from build123d import *

# Parameters (mm, degrees)
F1_DEPTH = 70
F2_R     = 5
F4_D     = 4
F4_DEPTH = 10
F4_TIP   = 1.2017212381


with BuildPart() as f1:
    # F0 (on Front) → F1 (new body)
    with BuildSketch(Plane.XZ):
        Polygon((3, 70), (0, 0), (18.5, 0), (18.5, 70), align=None)
    extrude(amount=F1_DEPTH)

    # F2
    f2_edges = [f1.edges().sort_by_distance(p)[0] for p in [
        (18.5, -35, 70),
        (3, -35, 70),
    ]]
    fillet(f2_edges, radius=F2_R)

    # F4
    with Locations(Plane(origin=(0, 0, 0), x_dir=(1, 0, 0), z_dir=(0, 0, -1))):
        with Locations((9.25, 55), (9.25, 15)):
            Hole(F4_D / 2, depth=F4_DEPTH)
            with Locations((0, 0, -(F4_DEPTH + F4_TIP / 2))):  # 118° drill point
                Cone(0, F4_D / 2, F4_TIP, mode=Mode.SUBTRACT)


solid = f1.part
Could you check a few things on this model? Use its own coordinates, in mm. A direction names the side the tool comes from. Give positions to 0.01 mm unless a question says otherwise; leave off trailing zeros. Order: outer loops, then holes, each group sorted by start corner. A loop starts at its lowest first (then second) coordinate and runs counter-clockwise, first axis right, second up.
1. Suppose I cut it at A-A (y = -29). Write out the boundary of the cut face in (x, z).
Answers below:
outline: (0, 0) - (18.5, 0) - (18.5, 65) arc R5 ccw to (13.5, 70) - (7.79, 70) arc R5 ccw to (2.79, 65.21) - close
2. Suppose I cut it at C-C (z = 17.5). Write out the boundary of the cut face in (x, y).
Answers below:
outline: (0.75, -70) - (18.5, -70) - (18.5, 0) - (0.75, 0) - close
3. Suppose I cut it at D-D (z = 53). Write out the boundary of the cut face in (x, y).
Answers below:
outline: (2.27, -70) - (18.5, -70) - (18.5, 0) - (2.27, 0) - close
4. Thinking about a two-plate mould opening in Y: for faces 1 (the flat face through (9, -70, 35)), 2 (the conical face through (9.4, -55.3, 11)), 3 (the cylindrical face through (4.29, -35.49, 68.57)), which applies, +Y half, -Y half, draft (parallel to the pull), parting line (faces both ways), or undercut?
Answers below:
face 1: -Y half
face 2: undercut
face 3: draft
5. For pin 1 (10 mm diameter, centred on y = -59.5, z = 33, fed in from -X); pin 2 (10 mm diameter, centred on x = 7.5, z = 18, fed in from +Y), each with a flat end and sliding along its axis, tell me the tip position at first contact or that it passes through.
Answers below:
pin 1: stops at x = 1.2
pin 2: stops at y = 0
6. Suppose I cut it at B-B (z = 6). Write out the boundary of the cut face in (x, y), plus the area to 3 significant figures.
Answers below:
outline: (0.26, -70) - (18.5, -70) - (18.5, 0) - (0.26, 0) - close; hole circle Ø4 at (9.25, -55); hole circle Ø4 at (9.25, -15)
area: 1,250 mm2
7. I need wall thicknesses on L1, parallel to Y at x = 9.25, z = 3.75; L2, parallel to X at y = -15, z = 6.75; L3, parallel to X at y = -15, z = 3. Which ranges of each line are inside material? Lowest first, please.
Answers below:
L1: y = -70 to -57, -53 to -17, -13 to 0
L2: x = 0.29 to 7.25, 11.25 to 18.5
L3: x = 0.13 to 7.25, 11.25 to 18.5
8. Which directions (+Z, -Z, +X, -X, +Y, -Y) give clear straight access to the entire face, cutting with the end or side of a thin tool? Please do faces 4 (the flat face through (18.5, -35, 32)), 5 (the cylindrical face through (9.51, -56.983, 5.07)).
Answers below:
face 4: +Z, -Z, +X, +Y, -Y
face 5: -Z
